Autodesk Inventor part; units mm, degrees
ref_plane "YZ Plane" through (0, 0, 0) normal (1, 0, 0) x (0, 1, 0)
ref_plane "XZ Plane" through (0, 0, 0) normal (0, 1, 0) x (-1, 0, 0)
ref_plane "XY Plane" through (0, 0, 0) normal (0, 0, 1) x (1, 0, 0)
sketch "Boceto1" plane through (0, 0, 0) normal (0, 1, 0) x (-1, 0, 0)
  line L0 (10.3005, 0.2018) -> (-1.6995, 0.2018)
  line L1 (-1.6995, 0.2018) -> (-1.6995, 18.2018)
  line L2 (-1.6995, 18.2018) -> (10.3005, 18.2018)
  line L3 (12.3005, 20.2018) -> (-3.6995, 20.2018)
  line L4 (-3.6995, 20.2018) -> (-3.6995, -1.7982)
  line L5 (-3.6995, -1.7982) -> (12.3005, -1.7982)
  line L6 (10.3005, 18.2018) -> (12.3005, 18.2018)
  line L7 (10.3005, 0.2018) -> (12.3005, 0.2018)
  line L8 (12.3005, -1.7982) -> (12.3005, 0.2018)
  line L9 (12.3005, 18.2018) -> (12.3005, 20.2018)
  point P0 (0, 0)
  dimension "d0" = 18
  dimension "d1" = 12
extrude "Extrusión1" add sketch "Boceto1" along normal blind 25
sketch "Boceto2" plane through (-12.3005, 0, 20.2018) normal (0, 0, 1) x (1, 0, 0)
  line L0 (16, 0) -> (16, 25)
  line L1 (0, 0) -> (14, 0)
  arc A0 (0, 0) -> (16, 0) centre (8, 0) ccw
  line L2 (0, 0) -> (16, 0)
sketch "Boceto3" plane through (3.6995, 0, -1.7982) normal (0, 0, -1) x (-1, 0, 0)
  line L0 (0, 0) -> (0, 25)
  line L1 (16, 0) -> (16, 25)
  arc A0 (0, 0) -> (16, 0) centre (8, -0.0367) ccw
  line L2 (16, 0) -> (0, 0)
  line L3 (16, 0) -> (2, 0)
  point P0 (3.6995, 0)
extrude "Extrusión2" add sketch "Boceto3" against normal blind 1
extrude "Extrusión3" add sketch "Boceto2" against normal blind 1
sketch "Boceto5" plane through (3.6995, 25, -1.7982) normal (0, 0, -1) x (-1, 0, 0)
  line L0 (0, 0) -> (16, 0)
  line L1 (16, -25) -> (16, 0)
  line L2 (16, 0) -> (0, 0)
  line L3 (16, 0) -> (16, -1.5)
  line L4 (16, 0) -> (0, 0)
  line L5 (0, -25) -> (0, 0)
  line L6 (0, 0) -> (0, -1.5)
  arc A0 (0.0504, -2.3965) -> (15.9464, -2.4245) centre (8, -1.5) ccw
  line L7 (15.9464, -2.4245) -> (15.9666, -2.3645)
  arc A1 (16, -2.3216) -> (15.9666, -2.3645) centre (16.045, -2.3909) ccw
  line L8 (0.0504, -2.3965) -> (0.0316, -2.3763)
  arc A2 (0.0316, -2.3763) -> (0, -2.3536) centre (-0.0406, -2.4434) ccw
  line L9 (16, -2.3216) -> (16, -1.5)
  line L10 (0, -1.5) -> (0, -2.3536)
  point P0 (3.6995, -25)
  dimension "d13" = 1.5
sketch "Boceto6" plane through (-12.3005, 25, 20.2018) normal (0, 0, 1) x (1, 0, 0)
  line L0 (16, 0) -> (0, 0)
  line L1 (16, -25) -> (16, 0)
  line L2 (0, 0) -> (16, 0)
  line L3 (0, 0) -> (0, -1.5)
  line L4 (0, -25) -> (0, 0)
  arc A0 (0.0942, -2.7242) -> (15.9182, -2.6413) centre (8, -1.5) ccw
  line L5 (16, -1.5) -> (16, 0)
  line L6 (15.9182, -2.6413) -> (15.9286, -2.6198)
  arc A1 (16, -2.5333) -> (15.9286, -2.6198) centre (16.1434, -2.7242) ccw
  line L7 (0.0942, -2.7242) -> (0.0677, -2.6601)
  arc A2 (0.0677, -2.6601) -> (0, -2.5946) centre (-0.0415, -2.7053) ccw
  line L8 (16, -2.5333) -> (16, 0)
  line L9 (0, -2.5946) -> (0, 0)
  point P0 (12.3005, -25)
  dimension "d10" = 1.5
extrude "Extrusión4" cut sketch "Boceto6" against normal blind 1
extrude "Extrusión5" cut sketch "Boceto5" against normal blind 1
sketch "Boceto8" plane through (-4.3005, -0.0367, -1.7982) normal (0, 0, -1) x (-1, 0, 0)
  circle A0 centre (0.1375, 20.0367) radius 1.75
  circle A1 centre (0.0632, -1.9632) radius 1.75
  line L0 (-8, 25.0367) -> (8, 25.0367)
  point P0 (-4.3005, 0.0367)
  dimension "d19" = 3.5
  dimension "d20" = 3.5
  dimension "d21" = 22
  dimension "d22" = 5
extrude "Extrusión6" add sketch "Boceto8" against normal blind 1 contours A0
extrude "Extrusión7" cut sketch "Boceto8" against normal blind 30 contours A1
sketch "Boceto9" plane through (-12.3005, 25, 19.2018) normal (0, 0, 1) x (1, 0, 0)
  circle A0 centre (7.8625, -5) radius 1.75
  circle A1 centre (7.8625, -5) radius 1.75
  point P0 (12.3005, -25)
extrude "Extrusión8" add sketch "Boceto9" along normal blind 1
sketch "Boceto10" plane through (-12.3005, 0, 0.2018) normal (-1, 0, 0) x (0, 0, 1)
  line L0 (-2, 0) -> (-2, 22.6784)
  line L1 (20, 0) -> (20, 22.4054)
  line L2 (0, 14.992) -> (18, 14.992)
  line L3 (0, 6.992) -> (18, 6.992)
  line L4 (0, 0) -> (0, 25)
  line L5 (0, 6.992) -> (0, 14.992)
  line L6 (18, 0) -> (18, 25)
  line L7 (18, 6.992) -> (18, 14.992)
  point P0 (-0.2018, 0)
  dimension "d32" = 8
extrude "Extrusión9" add sketch "Boceto10" against normal blind 1
sketch "Boceto11" plane through (3.6995, 0, -0.7982) normal (1, 0, 0) x (0, 0, -1)
  point P0 (-0.7982, 0)
sketch "Boceto12" plane through (1.6995, 0, 0.2018) normal (-1, 0, 0) x (0, 0, 1)
  line L0 (0, 14.992) -> (0, 25)
  line L1 (0, 25) -> (0, 20)
  line L2 (0, 20) -> (18, 20)
  line L3 (18, 14.992) -> (18, 25)
  line L4 (18, 25) -> (0, 25)
  line L5 (19, 25) -> (-1, 25)
  line L6 (18, 25) -> (18, 20)
  line L7 (-1, 0) -> (0, 0)
  line L8 (0, 0) -> (0, 4)
  line L9 (0, 0) -> (0, 25)
  line L10 (0, 4) -> (18, 4)
  line L11 (18, 0) -> (18, 25)
  line L12 (0, 0) -> (18, 0)
  line L13 (18, 4) -> (18, 0)
  line L14 (18, 0) -> (0, 0)
  point P0 (-0.2018, 0)
  dimension "d35" = 5
  dimension "d36" = 4
extrude "Extrusión10" cut sketch "Boceto12" against normal blind 2 contours L0 L4 L3 L2 | L10 L11 L12 L8
properties part number "Eslabon cadena portacable"
CAD build for the part. Positions are in the model's coordinates, mm. A direction names the side the tool comes from. Round coordinates to 2 decimals unless told otherwise and drop trailing zeros. Order: outer loops, then holes, each group sorted by start corner. A loop starts at its lowest first (then second) coordinate and runs counter-clockwise, first axis right, second up.
Item 1: Probe line 1 along Z through (x, y) = (2.75, 0.5); line 2 along Z through (x, y) = (1.25, 19); line 3 along X through (y, z) = (10.5, 12). List the from-to ranges inside material, lowest first.
Item 2: Mould opens along Z. For faces 1 (the face through (3, 4, 9)), 2 (the face through (-2.615, -1.923, -1.305)), 3 (the face through (-4, 22, 19.202)) say: pulls with the +Z half, pulls with the -Z half, needs draft (parallel to the pull), parting line crosses it, or undercut.
Item 3: Saw through at C-C on y = 10. Write the cut outline in (x, z).
Item 4: Pin check, flat tips, straight feed: pin 1 (6 mm diameter, centred on x = -0.5, z = 1.5, fed in from -Y); pin 2 (1.6 mm diameter, centred on x = 3, z = 6.5, fed in from +Y); pin 3 (3 mm diameter, centred on x = -4.36, y = -2, fed in from -Z) (1 decimal); pin 4 (0.5 mm diameter, centred on x = -12, z = 12.5, fed in from +Y). Stop position of each tip, or through.
Item 5: Saw through at B-B on y = 3. Write the cut outline in (x, z), then the cut area to 3 significant figures.
Item 6: Tool access for faces 4 (the face through (-12, 14.992, 9)), 5 (the face through (1.7, 12, 9)), 6 (the face through (-4.666, 18.265, 19.695)), 7 (the face through (-4, -4, 19.202)), 8 (the face through (3, 20, 9)): list every direction of +Z, -Z, +X, -X, +Y, -Y with a clear straight run to the whole face (end or side of a thin tool).
Item 7: Saw through at A-A on z = 15.5. Write the cut outline in (x, y).
Item 8: Saw through at D-D on x = -3.25. State how many separate pieces and enclosed holes the cut face has, then the cut area to 3 significant figures.
Reported:
1. line 1: z = -1.8 to 0.2, 18.2 to 20.2
1. line 2: z = -0.8 to 0.2, 18.2 to 19.2
1. line 3: x = -12.3 to -11.3, 1.7 to 3.7
2. face 1: undercut
2. face 2: needs draft
2. face 3: pulls with the +Z half
3. outline: (-12.3, -1.8) - (3.7, -1.8) - (3.7, 20.2) - (-12.3, 20.2) - close; hole (-11.3, 0.2) - (1.7, 0.2) - (1.7, 18.2) - (-11.3, 18.2) - close
4. pin 1: stops at y = -7.81
4. pin 2: stops at y = 20
4. pin 3: passes through
4. pin 4: stops at y = 14.99
5. outline: (-12.3, -1.8) - (3.7, -1.8) - (3.7, 0.2) - (-12.3, 0.2) - close; (-12.3, 18.2) - (3.7, 18.2) - (3.7, 20.2) - (-12.3, 20.2) - close
5. area: 64.0 mm2
6. face 4: -X, +Y
6. face 5: +Y, -Y
6. face 6: +Z
6. face 7: +X, -X, -Y
6. face 8: +X, -X, +Y
7. outline: (-12.3, 6.99) - (-11.3, 6.99) - (-11.3, 14.99) - (-12.3, 14.99) - close; (1.7, 4) - (3.7, 4) - (3.7, 20) - (1.7, 20) - close
8. separate pieces: 4
8. enclosed holes: 0
8. area: 96.8 mm2
